Could you check a few things on this drawing? It's one solid part, dimensions in mm from its lowest x, y, z. Round coordinates to 2 decimals unless told otherwise and drop trailing zeros. Write each loop counter-clockwise with the first axis right and the second up, starting at its lowest first coordinate (ties: lowest second). Pieces come first, ordered by that corner, then holes. Notation, with made-up numbers: (11.5, -15) -> (23.5, -15) arc R25 ccw to (23.5, 8) -> close; hole circle Ø3 at (43.5, 41.25). An arc over 180 degrees is marked (long way). Answer as CSV lines item,"result".
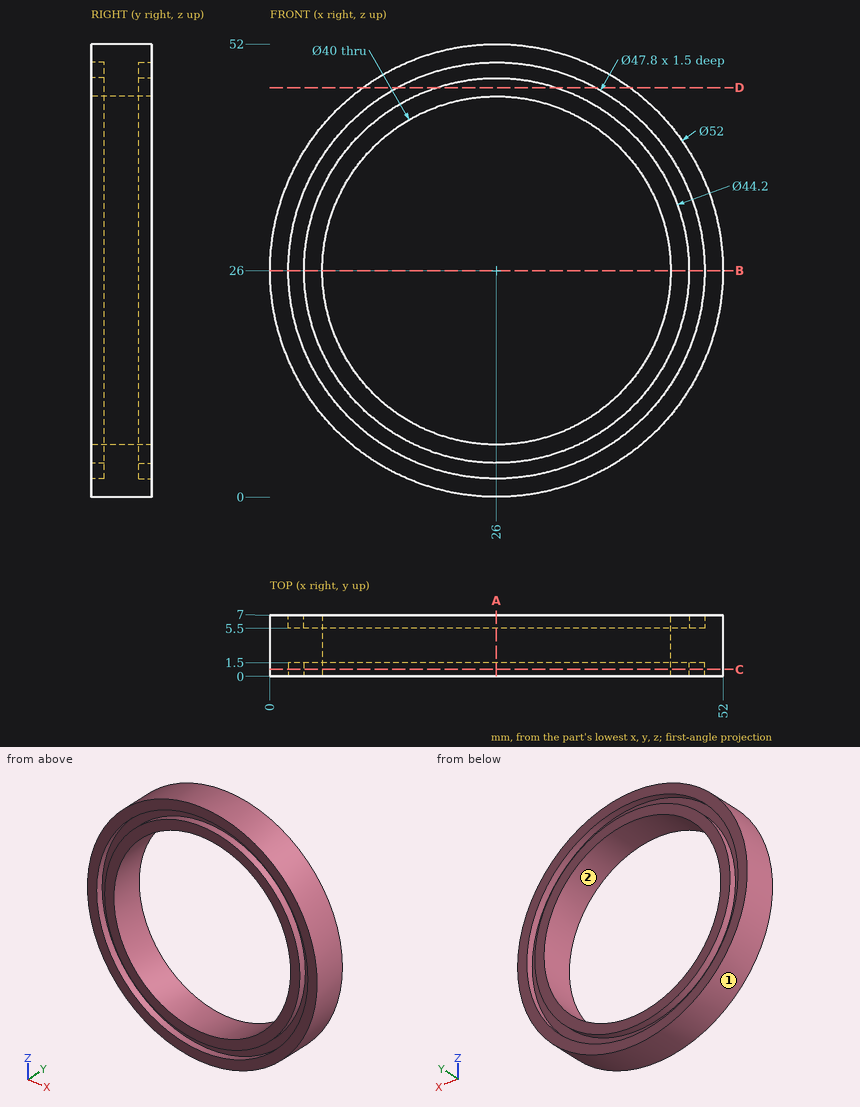
1. Suppose I cut it at D-D on z = 47. Please give me the cut outline in (x, y), and give its area (3 significant figures).
Numbers:
outline,"(10.67, 0) -> (14.59, 0) -> (14.59, 1.5) -> (19.11, 1.5) -> (19.11, 0) -> (32.89, 0) -> (32.89, 1.5) -> (37.41, 1.5) -> (37.41, 0) -> (41.33, 0) -> (41.33, 7) -> (37.41, 7) -> (37.41, 5.5) -> (32.89, 5.5) -> (32.89, 7) -> (19.11, 7) -> (19.11, 5.5) -> (14.59, 5.5) -> (14.59, 7) -> (10.67, 7) -> close"
area,"187 mm^2"
2. Suppose I cut it at C-C on y = 0.75. Please give me the cut outline in (x, z), and give its area (3 significant figures).
Numbers:
outline,"circle Ø52 at (26, 26); circle Ø44.2 at (26, 26); hole circle Ø47.8 at (26, 26); hole circle Ø40 at (26, 26)"
area,"607 mm^2"
3. If I drill on line 1 (X direction, y = 6.05, z = 26); line 2 (X direction, y = 5, z = 26), over which ranges is the centre line in solid material (lowest first)?
Numbers:
line 1,"x = 0 to 2.1, 3.9 to 6, 46 to 48.1, 49.9 to 52"
line 2,"x = 0 to 6, 46 to 52"
4. For pin 1 Ø1 at (x, y) = (30, 4.5) entering from -Z; pin 2 Ø1 at (y, z) = (4, 21.5) entering from +X; pin 3 Ø2 at (x, y) = (35, 3) entering from -Z; pin 4 Ø24 at (x, z) = (17.5, 30.5) entering from -Y, each with a flat end and sliding along its axis, tell me the tip position at first contact or that it passes through.
Numbers:
pin 1,"stops at z = 0.24"
pin 2,"stops at x = 51.69"
pin 3,"stops at z = 1.26"
pin 4,"stops at y = 0"
5. Suppose I cut it at B-B on z = 26. Please give me the cut outline in (x, y), and give its area (3 significant figures).
Numbers:
outline,"(0, 0) -> (2.1, 0) -> (2.1, 1.5) -> (3.9, 1.5) -> (3.9, 0) -> (6, 0) -> (6, 7) -> (3.9, 7) -> (3.9, 5.5) -> (2.1, 5.5) -> (2.1, 7) -> (0, 7) -> close; (46, 0) -> (48.1, 0) -> (48.1, 1.5) -> (49.9, 1.5) -> (49.9, 0) -> (52, 0) -> (52, 7) -> (49.9, 7) -> (49.9, 5.5) -> (48.1, 5.5) -> (48.1, 7) -> (46, 7) -> close"
area,"73.2 mm^2"
6. Suppose I cut it at A-A on x = 26. Please give me the cut outline in (y, z).
Numbers:
outline,"(0, 0) -> (7, 0) -> (7, 2.1) -> (5.5, 2.1) -> (5.5, 3.9) -> (7, 3.9) -> (7, 6) -> (0, 6) -> (0, 3.9) -> (1.5, 3.9) -> (1.5, 2.1) -> (0, 2.1) -> close; (0, 46) -> (7, 46) -> (7, 48.1) -> (5.5, 48.1) -> (5.5, 49.9) -> (7, 49.9) -> (7, 52) -> (0, 52) -> (0, 49.9) -> (1.5, 49.9) -> (1.5, 48.1) -> (0, 48.1) -> close"
7. If we mould it in two halves opening along Z, with no side actions, what happens to the marked faces 1 and 2? For each: released by +Z, released by -Z, zero draft, split by the parting line, or undercut.
Numbers:
face 1,"split by the parting line"
face 2,"undercut"
